```python
from build123d import *

# Parameters (mm, degrees)
BOSS_EXTRUDE1_DEPTH     = 0.77
BOSS_EXTRUDE2_DEPTH     = 1
CUT_EXTRUDE1_DEPTH      = 55.235597166
CUT_EXTRUDE1_DEPTH_BACK = 55.235597166
CHAMFER1_SIZE           = 0.25


with BuildPart() as part:
    # Sketch2 → Boss-Extrude1 (new body)
    with BuildSketch(Plane.ZY):
        with BuildLine():
            Line((-27.5, 41), (-27.5, -41))
            ThreePointArc((-27.5, -41), (-26.767766953, -42.767766953), (-25, -43.5))
            Line((-25, -43.5), (25, -43.5))
            ThreePointArc((25, -43.5), (26.767766953, -42.767766953), (27.5, -41))
            Line((27.5, -41), (27.5, 41))
            ThreePointArc((27.5, 41), (26.767766953, 42.767766953), (25, 43.5))
            Line((25, 43.5), (-25, 43.5))
            ThreePointArc((-25, 43.5), (-26.767766953, 42.767766953), (-27.5, 41))
        make_face()
    extrude(amount=-BOSS_EXTRUDE1_DEPTH)

    # Sketch3 → Boss-Extrude2 (add)
    with BuildSketch(Plane.ZY):
        with BuildLine():
            Line((-29.5, 41), (-29.5, -41))
            ThreePointArc((-29.5, -41), (-28.181980515, -44.181980515), (-25, -45.5))
            Line((-25, -45.5), (25, -45.5))
            ThreePointArc((25, -45.5), (28.181980515, -44.181980515), (29.5, -41))
            Line((29.5, -41), (29.5, 41))
            ThreePointArc((29.5, 41), (28.181980515, 44.181980515), (25, 45.5))
            Line((25, 45.5), (-25, 45.5))
            ThreePointArc((-25, 45.5), (-28.181980515, 44.181980515), (-29.5, 41))
        make_face()
    extrude(amount=BOSS_EXTRUDE2_DEPTH)

    # Sketch3<3> → Cut-Extrude1 (cut, two sides: drawn at the far end of the back side and taken through both)
    with BuildSketch(Plane.ZY.offset(-CUT_EXTRUDE1_DEPTH_BACK)):
        with BuildLine():
            Line((25, 41.999999952), (-25, 41.999999952))
            ThreePointArc((-25, 41.999999952), (-25.707106747, 41.707106747), (-25.999999952, 41))
            Line((-25.999999952, 41), (-25.999999952, -41))
            ThreePointArc((-25.999999952, -41), (-25.707106747, -41.707106747), (-25, -41.999999952))
            Line((-25, -41.999999952), (25, -41.999999952))
            ThreePointArc((25, -41.999999952), (25.707106747, -41.707106747), (25.999999952, -41))
            Line((25.999999952, -41), (25.999999952, 41))
            ThreePointArc((25.999999952, 41), (25.707106747, 41.707106747), (25, 41.999999952))
        make_face()
    extrude(amount=CUT_EXTRUDE1_DEPTH + CUT_EXTRUDE1_DEPTH_BACK, mode=Mode.SUBTRACT)

    # Chamfer1
    chamfer1_edges = [part.edges().sort_by_distance(p)[0] for p in [
        (0.77, -43.5, 0),
        (0.77, -42.767766953, 26.767766953),
        (0.77, 0, 27.5),
        (0.77, 42.767766953, 26.767766953),
        (0.77, 43.5, 0),
        (0.77, 42.767766953, -26.767766953),
        (0.77, 0, -27.5),
        (0.77, -42.767766953, -26.767766953),
    ]]
    chamfer(chamfer1_edges, length=CHAMFER1_SIZE)


solid = part.part
```
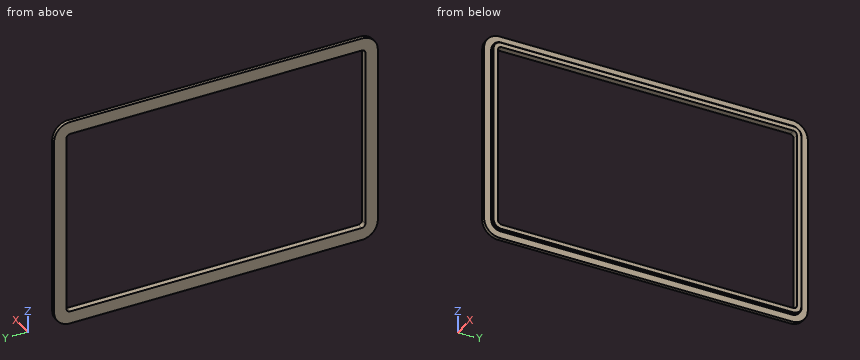
Build history of the part. All positions in model axes, mm. Round coordinates to 2 decimals unless told otherwise and drop trailing zeros. Order: outer loops, then holes, each group sorted by start corner. A loop starts at its lowest first (then second) coordinate and runs counter-clockwise, first axis right, second up. Notation, with made-up numbers: (67, 63.25) -> (79, 63.25) arc R33 ccw to (79, 96.25) -> close; hole circle Ø10 at (-14, -29). An arc over 180 degrees is marked (long way). Answer in a Markdown table with one row per item.
1) Band-saw the part on A-A on z = 19. Give the cut face in (x, y).
Values:
| item | result |
|---|---|
| outline | (-1, -45.5) -> (0, -45.5) -> (0, -43.5) -> (0.52, -43.5) -> (0.77, -43.25) -> (0.77, -42) -> (-1, -42) -> close; (-1, 42) -> (0.77, 42) -> (0.77, 43.25) -> (0.52, 43.5) -> (0, 43.5) -> (0, 45.5) -> (-1, 45.5) -> close |
2) Wall check: L1, parallel to Y at x = -0.5, z = 11; L2, parallel to Z at x = -0.5, y = -31; L3, parallel to Y at x = 0.4, z = -9. Give the ranges that are in metal, low to high.
Values:
| item | result |
|---|---|
| L1 | -45.5 to -42, 42 to 45.5 |
| L2 | -29.5 to -26, 26 to 29.5 |
| L3 | -43.5 to -42, 42 to 43.5 |
3) Band-saw the part on B-B on y = 6.5. Give the cut face in (x, z), and give its area (3 significant figures).
Values:
| item | result |
|---|---|
| outline | (-1, -29.5) -> (0, -29.5) -> (0, -27.5) -> (0.52, -27.5) -> (0.77, -27.25) -> (0.77, -26) -> (-1, -26) -> close; (-1, 26) -> (0.77, 26) -> (0.77, 27.25) -> (0.52, 27.5) -> (0, 27.5) -> (0, 29.5) -> (-1, 29.5) -> close |
| area | 9.25 mm2 |
